Autodesk Inventor part; units mm, degrees
ref_plane "YZ Plane" through (0, 0, 0) normal (1, 0, 0) x (0, 1, 0)
ref_plane "XZ Plane" through (0, 0, 0) normal (0, 1, 0) x (-1, 0, 0)
ref_plane "XY Plane" through (0, 0, 0) normal (0, 0, 1) x (1, 0, 0)
sketch "Szkic1" plane through (0, 0, 0) normal (0, 1, 0) x (-1, 0, 0)
  line L0 (34.8855, -22.7009) -> (-28.1145, -22.7009)
  line L1 (-28.1145, -22.7009) -> (-28.1145, -57.7009)
  line L2 (-28.1145, -57.7009) -> (34.8855, -57.7009)
  line L3 (34.8855, -57.7009) -> (34.8855, -22.7009)
  line L4 (-28.1145, -57.7009) -> (-8.1145, -57.7009)
  line L5 (-8.1145, -57.7009) -> (-8.1145, 45.2991)
  line L6 (-8.1145, 45.2991) -> (-28.1145, 45.2991)
  line L7 (-28.1145, 45.2991) -> (-28.1145, -57.7009)
  point P0 (0, 0)
  point P1 (-8.1145, -22.7009)
  dimension "d0" = 63
  dimension "d1" = 35
  dimension "d2" = 103
  dimension "d3" = 20
extrude "Wyciągnięcie proste1" add sketch "Szkic1" along normal blind 4
properties part number "S5_Mainboard"
Input: part model. Units: mm. Frame: model coordinates. A direction names the side the tool comes from. Coordinates: 2 decimals unless noted, no trailing zeros. Order: outer loops, then holes, each group sorted by start corner. A loop starts at its lowest first (then second) coordinate and runs counter-clockwise, first axis right, second up.
1. Cut plane B-B, the plane y = 1.7. Return loops of the section in (x, z), plus the area to 4 significant figures.
Checked values:
outline: (-34.89, -57.7) - (28.11, -57.7) - (28.11, 45.3) - (8.11, 45.3) - (8.11, -22.7) - (-34.89, -22.7) - close
area: 3,565 mm2
2. Cut plane A-A, the plane z = -13. Return loops of the section in (x, y), plus the area to 3 significant figures.
Checked values:
outline: (8.11, 0) - (28.11, 0) - (28.11, 4) - (8.11, 4) - close
area: 80.0 mm2
3. Cut plane C-C, the plane x = 3.5. Return loops of the section in (y, z).
Checked values:
outline: (0, -57.7) - (4, -57.7) - (4, -22.7) - (0, -22.7) - close
4. Access query for faces 1 (the flat face through (-14, 2, -22.701)), 2 (the flat face through (-3, 2, -57.701)). Directions: +Z, -Z, +X, -X, +Y, -Y. A direction counts if a zero-diameter tool reaches every point of the face in a straight line with its end or side. Return the directions, or none.
Checked values:
face 1: +Z, -X, +Y, -Y
face 2: -Z, +X, -X, +Y, -Y
5. Ray query, line 1 along Z through (x, y) = (-16, 0.4); line 2 along X through (y, z) = (0.3, -1). Return the intervals inside material, ascending.
Checked values:
line 1: z = -57.7 to -22.7
line 2: x = 8.11 to 28.11
